Could you check a few things on this model? Use its own coordinates, in mm. A direction names the side the tool comes from. Coordinates: 2 decimals unless noted, no trailing zeros. Write each loop counter-clockwise with the first axis right and the second up, starting at its lowest first coordinate (ties: lowest second). Pieces come first, ordered by that corner, then holes. Notation, with made-up numbers: (1, 32.25) - (33, 32.25) arc R36 cw to (33, 68.25) - close; hole circle Ø7 at (-19.5, -11). An arc over 180 degrees is marked (long way). Answer as a JSON object with one key per item and string values. Group by question number.
1) Please list where these lines run through material, in increasing order: line 1 along Z through (x, y) = (-7, -3.25); line 2 along Y through (x, z) = (-10.95, -7); line 3 along X through (y, z) = (0.25, 4.75).
2) If we section it at A-A (x = -10.95): Write out the boundary of the cut face in (y, z).
3) On a 3-axis mill with a long thin cutter (end or side, diameter ignored), from which of +Z, -Z, +X, -X, +Y, -Y can I reach the whole of each face in a straight line? I mean faces 5 (the flat face through (-6.45, 0, 0)), 6 (the flat face through (3, 6.25, 0)). Say none if no direction works.
4) Will this pin go through, and if not, where does the flat tip stop? pin 1 Ø4 at (x, y) = (-10.95, -1.17) entering from +Z.
5) We'd pull the mould along Z, two halves only. Please class faces 1 (the flat face through (-11, 1.5, -6)), 2 (the cylindrical face through (-8.8, -0.5, -7.7)), 3 (the flat face through (0, 0, 9.5)), 4 (the flat face through (0, 0, -9.5)): released by +Z, released by -Z, zero draft, split by the parting line, or undercut.
6) If we section it at D-D (y = -1.17): Write out the boundary of the cut face in (x, z), plus the area to 3 significant figures.
7) If we section it at C-C (y = -4.25): Write out the boundary of the cut face in (x, z).
8) If we section it at B-B (y = 0.75): Write out the boundary of the cut face in (x, z), plus the area to 3 significant figures.
```python
from build123d import *

# Parameters (mm, degrees)
SKETCH1_W           = 30.9
SKETCH1_H           = 12.5
BOSS_EXTRUDE1_DEPTH = 9.499999986
SKETCH2_W           = 9
SKETCH2_H           = 12
CUT_EXTRUDE1_DEPTH  = 12.5
SKETCH3_R           = 2.25
CUT_EXTRUDE2_DEPTH  = 19


with BuildPart() as part:
    # Sketch1 → Boss-Extrude1 (new body, symmetric)
    with BuildSketch(Plane.XY):
        Rectangle(SKETCH1_W, SKETCH1_H)
    extrude(amount=BOSS_EXTRUDE1_DEPTH, both=True)

    # Sketch2 → Cut-Extrude1 (cut)
    with BuildSketch(Plane(origin=(0, 6.25, 0), x_dir=(1, 0, 0), z_dir=(0, 1, 0))):
        with Locations((-10.95, 0)):
            Rectangle(SKETCH2_W, SKETCH2_H)
    extrude(amount=-CUT_EXTRUDE1_DEPTH, mode=Mode.SUBTRACT)

    # Sketch3 → Cut-Extrude2 (cut)
    with BuildSketch(Plane.XY.offset(9.499999986)):
        with Locations((-10.95, -1.17)):
            Circle(SKETCH3_R)
    extrude(amount=-CUT_EXTRUDE2_DEPTH, mode=Mode.SUBTRACT)


solid = part.part
```
Here are the results:
{
 "1": {"line 1": "z = -9.5 to -6, 6 to 9.5", "line 2": "y = -6.25 to -3.42, 1.08 to 6.25", "line 3": "x = -6.45 to 15.45"},
 "2": {"outline": "(-6.25, -9.5) - (-3.42, -9.5) - (-3.42, -6) - (-6.25, -6) - close; (-6.25, 6) - (-3.42, 6) - (-3.42, 9.5) - (-6.25, 9.5) - close; (1.08, -9.5) - (6.25, -9.5) - (6.25, -6) - (1.08, -6) - close; (1.08, 6) - (6.25, 6) - (6.25, 9.5) - (1.08, 9.5) - close"},
 "3": {"face 5": "-X, +Y, -Y", "face 6": "+Z, -Z, +X, -X, +Y"},
 "4": {"pin 1": "passes through"},
 "5": {"face 1": "undercut", "face 2": "zero draft", "face 3": "released by +Z", "face 4": "released by -Z"},
 "6": {"outline": "(-15.45, -9.5) - (-13.2, -9.5) - (-13.2, -6) - (-15.45, -6) - close; (-15.45, 6) - (-13.2, 6) - (-13.2, 9.5) - (-15.45, 9.5) - close; (-8.7, -9.5) - (15.45, -9.5) - (15.45, 9.5) - (-8.7, 9.5) - (-8.7, 6) - (-6.45, 6) - (-6.45, -6) - (-8.7, -6) - close", "area": "448 mm²"},
 "7": {"outline": "(-15.45, -9.5) - (15.45, -9.5) - (15.45, 9.5) - (-15.45, 9.5) - (-15.45, 6) - (-6.45, 6) - (-6.45, -6) - (-15.45, -6) - close"},
 "8": {"outline": "(-15.45, -9.5) - (-12.12, -9.5) - (-12.12, -6) - (-15.45, -6) - close; (-15.45, 6) - (-12.12, 6) - (-12.12, 9.5) - (-15.45, 9.5) - close; (-9.78, -9.5) - (15.45, -9.5) - (15.45, 9.5) - (-9.78, 9.5) - (-9.78, 6) - (-6.45, 6) - (-6.45, -6) - (-9.78, -6) - close", "area": "463 mm²"}
}
